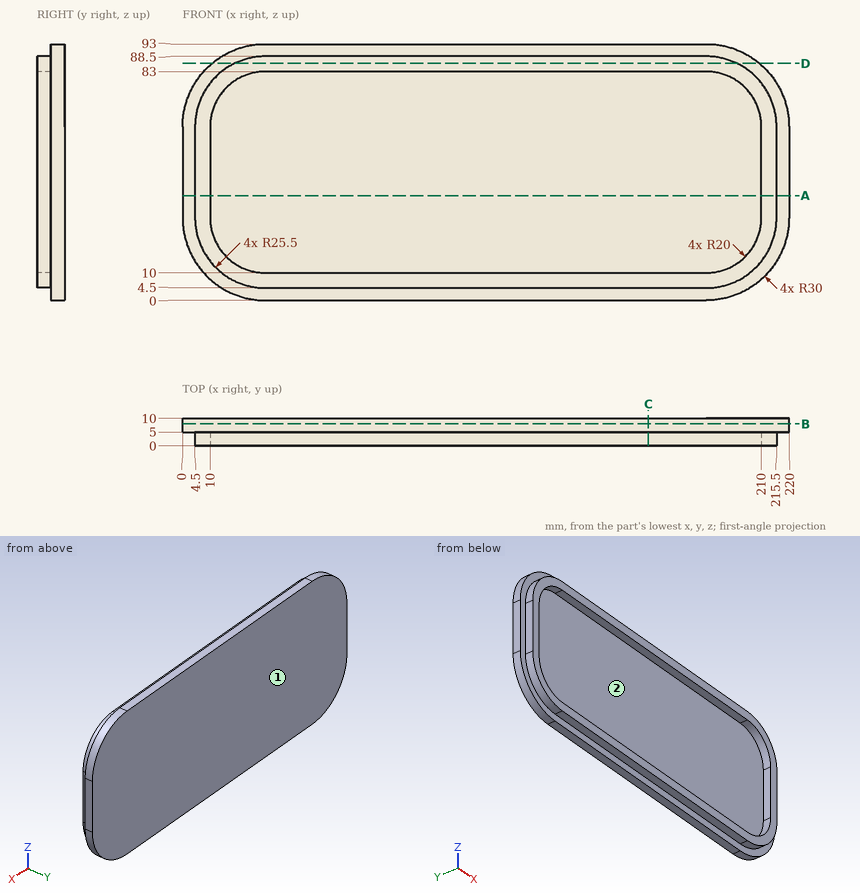
Check sheet for the drawn part. Datum: minimum x, y, z corner. Units: mm. Coordinates: 2 decimals unless noted, no trailing zeros. Order: outer loops, then holes, each group sorted by start corner. A loop starts at its lowest first (then second) coordinate and runs counter-clockwise, first axis right, second up. Notation, with made-up numbers: (70.5, 18) -> (118.5, 18) arc R20 ccw to (118.5, 25) -> close; hole circle Ø1 at (43, -36.75). An arc over 180 degrees is marked (long way). Write each question's results on one line, items separated by ' | '. Start each with the question number.
1) Draft check along X on the marked faces 1 and 2. Enter one of: pulls with the +X half, pulls with the -X half, needs draft (parallel to the pull), parting line crosses it, or undercut.
2) Depth check by flat-ended pin: pin 1 (1 mm diameter, centred on x = 138.5, y = 8.5, fed in from -Z); pin 2 (10 mm diameter, centred on x = 95, z = 30.5, fed in from -Y); pin 3 (2.5 mm diameter, centred on y = 2, z = 42.5, fed in from +X); pin 4 (1.5 mm diameter, centred on x = 112, y = 3.5, fed in from +Z). Enter the tip coordinate at first touch or a pass-through.
3) Section check C-C (x = 169). Enter the section's corners in (y, z), and give its area (3 significant figures).
4) Section check A-A (z = 38). Enter the section's corners in (x, y), and give its area (4 significant figures).
5) Section check D-D (z = 86). Enter the section's corners in (x, y), and give its area (3 significant figures).
6) Section check B-B (y = 8). Enter the section's corners in (x, z).
7) Material ranges on line 1 along Z through (x, y) = (138, 2); line 2 along X through (y, z) = (2.5, 39.5); line 3 along Y through (x, z) = (125, 56.5), recorded low to high.
Checked values:
1) face 1: needs draft | face 2: undercut
2) pin 1: z = 0 | pin 2: y = 5 | pin 3: x = 215.5 | pin 4: z = 88.5
3) outline: (0, 4.5) -> (5, 4.5) -> (5, 0) -> (10, 0) -> (10, 93) -> (5, 93) -> (5, 88.5) -> (0, 88.5) -> (0, 83) -> (5, 83) -> (5, 10) -> (0, 10) -> close | area: 520 mm²
4) outline: (0, 5) -> (4.5, 5) -> (4.5, 0) -> (10, 0) -> (10, 5) -> (210, 5) -> (210, 0) -> (215.5, 0) -> (215.5, 5) -> (220, 5) -> (220, 10) -> (0, 10) -> close | area: 1,155 mm²
5) outline: (10.74, 5) -> (18.99, 5) -> (18.99, 0) -> (201.01, 0) -> (201.01, 5) -> (209.26, 5) -> (209.26, 10) -> (10.74, 10) -> close | area: 1,900 mm²
6) outline: (0, 30) arc R30 ccw to (30, 0) -> (190, 0) arc R30 ccw to (220, 30) -> (220, 63) arc R30 ccw to (190, 93) -> (30, 93) arc R30 ccw to (0, 63) -> close
7) line 1: 4.5 to 10, 83 to 88.5 | line 2: 4.5 to 10, 210 to 215.5 | line 3: 5 to 10
